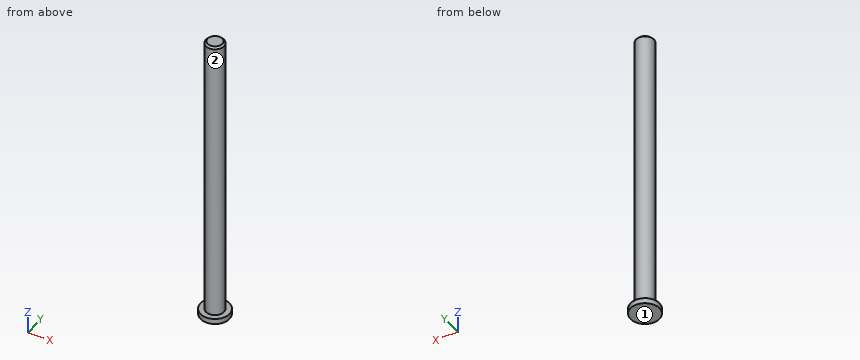
from build123d import *

# Parameters (mm, degrees)
SKETCH1_R           = 4
BOSS_EXTRUDE1_DEPTH = 1.5
SKETCH2_R           = 2.5
BOSS_EXTRUDE2_DEPTH = 80
CHAMFER1_SIZE       = 0.5


with BuildPart() as part:
    # Sketch1 → Boss-Extrude1 (new body)
    with BuildSketch(Plane.XY):
        Circle(SKETCH1_R)
    extrude(amount=BOSS_EXTRUDE1_DEPTH)

    # Sketch2 → Boss-Extrude2 (add)
    with BuildSketch(Plane.XY.offset(1.5)):
        Circle(SKETCH2_R)
    extrude(amount=BOSS_EXTRUDE2_DEPTH)

    # Chamfer1
    chamfer1_edges = [part.edges().sort_by_distance(p)[0] for p in [
        (-2.5, 0, 81.5),
    ]]
    chamfer(chamfer1_edges, length=CHAMFER1_SIZE)


solid = part.part
Input: part model. Units: mm. Frame: model coordinates. Face numbers are marked on the shaded views. A direction names the side the tool comes from. Round coordinates to 2 decimals unless told otherwise and drop trailing zeros. Order: outer loops, then holes, each group sorted by start corner. A loop starts at its lowest first (then second) coordinate and runs counter-clockwise, first axis right, second up. Notation, with made-up numbers: (84.5, 71.25) - (97.5, 71.25) arc R19 ccw to (97.5, 84.25) - close; hole circle Ø5 at (21.25, 72.5). An arc over 180 degrees is marked (long way). Use a Markdown table: item, result.
1. Access query for the marked faces 1 and 2. Directions: +Z, -Z, +X, -X, +Y, -Y. A direction counts if a zero-diameter tool reaches every point of the face in a straight line with its end or side. Return the directions, or none.
Evaluation:
| item | result |
|---|---|
| face 1 | -Z, +X, -X, +Y, -Y |
| face 2 | +Z |
2. Section A-A on x = 0. Return the cut outline in (y, z), then the cut area to 3 significant figures.
Evaluation:
| item | result |
|---|---|
| outline | (-4, 0) - (4, 0) - (4, 1.5) - (2.5, 1.5) - (2.5, 81) - (2, 81.5) - (-2, 81.5) - (-2.5, 81) - (-2.5, 1.5) - (-4, 1.5) - close |
| area | 412 mm^2 |
3. Material intervals for probe 1 along Z at (x, y) = (-1, 3.75); probe 2 along Z at (x, y) = (-1.75, -1); probe 3 along Y at (x, z) = (1.5, 63.5), sorted ascending.
Evaluation:
| item | result |
|---|---|
| probe 1 | 0 to 1.5 |
| probe 2 | 0 to 81.48 |
| probe 3 | -2 to 2 |
4. First-contact query: pin 1 (2 mm diameter, centred on x = 3, z = 53.5, fed in from -Y); pin 2 (4 mm diameter, centred on x = 1.5, y = -1.5, fed in from +Z); pin 3 (3 mm diameter, centred on y = -3, z = 40, fed in from +X); pin 4 (1.5 mm diameter, centred on y = 3, z = 63.5, fed in from +X). Flat tips, straight axial feed; report the tip coordinate or a pass-through.
Evaluation:
| item | result |
|---|---|
| pin 1 | y = -1.5 |
| pin 2 | z = 81.5 |
| pin 3 | x = 2 |
| pin 4 | x = 1.09 |
